Study the drawing (mm; zero at the part's minimum x, y, z) and answer. Coordinates: 2 decimals unless noted, no trailing zeros. Write each loop counter-clockwise with the first axis right and the second up, starting at its lowest first coordinate (ties: lowest second). Pieces come first, ordered by that corner, then holes. Notation, with made-up numbers: (84.5, 88.5) -> (117.5, 88.5) arc R18 ccw to (117.5, 92.5) -> close; hole circle Ø9 at (13, 5). An arc over 180 degrees is marked (long way). Answer in a Markdown table with one row per item. Add a question column.
Item 1: For a pull along X with two mould halves and no side action, classify the marked faces 1, 2 and 3 as +X half, -X half, draft (parallel to the pull), parting line (faces both ways), or undercut.
Item 2: Straight lines are drawn through the part: line 1 (Y direction, x = 6.5, z = 4.3) (1 decimal); line 2 (Y direction, x = 7.75, z = 2.7) (1 decimal); line 3 (X direction, y = 4, z = 4.3). For each, find the intervals that lie inside material, in ascending order. Write a range as from..to.
Item 3: Section D-D on x = 10 is taken. Write down the section's boundary in (y, z) (1 decimal).
Item 4: Section B-B on y = 4.25 is taken. Write down the section's boundary in (x, z) (1 decimal), then the cut area to 3 significant figures.
Item 5: Section A-A on x = 3.5 is taken. Write down the section's boundary in (y, z) (1 decimal).
Item 6: Given pin 1 Ø1 at (y, z) = (7.5, 2.5) entering from -X; pin 2 Ø1 at (x, z) = (4.5, 0.5) entering from +Y; pin 3 Ø4 at (x, y) = (5.58, 5.15) entering from -Z, each flat-ended and moving along its own axis, determine where each tip first touches the part or whether it passes through.
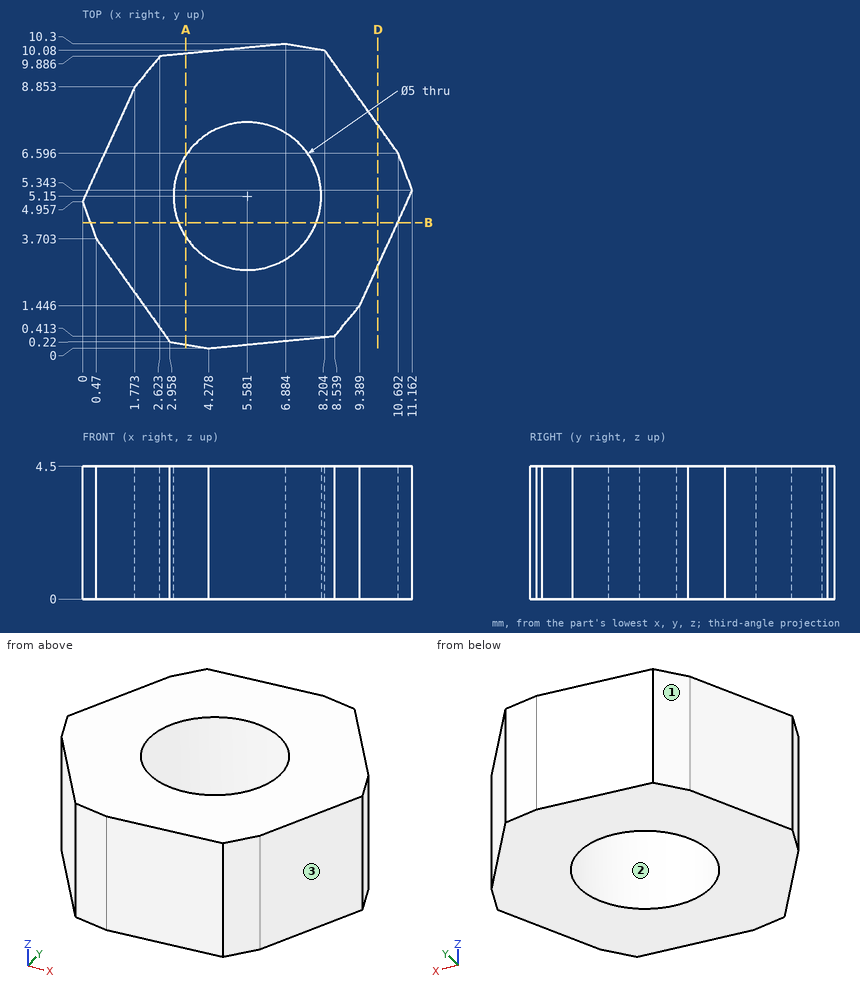
Results below:
| question | item | result |
|---|---|---|
| 1 | face 1 | -X half |
| 1 | face 2 | undercut |
| 1 | face 3 | +X half |
| 2 | line 1 | y = 0.2..2.8, 7.5..10.3 |
| 2 | line 2 | y = 0.3..3.9, 6.4..10.2 |
| 2 | line 3 | x = 0.36..3.36, 7.8..10.55 |
| 3 | outline | (2.8, 0) -> (7.6, 0) -> (7.6, 4.5) -> (2.8, 4.5) -> close |
| 4 | outline | (0.3, 0) -> (3.2, 0) -> (3.2, 4.5) -> (0.3, 4.5) -> close; (7.9, 0) -> (10.7, 0) -> (10.7, 4.5) -> (7.9, 4.5) -> close |
| 4 | area | 25.8 mm2 |
| 5 | outline | (0.1, 0) -> (3.8, 0) -> (3.8, 4.5) -> (0.1, 4.5) -> close; (6.5, 0) -> (10, 0) -> (10, 4.5) -> (6.5, 4.5) -> close |
| 6 | pin 1 | stops at x = 0.93 |
| 6 | pin 2 | stops at y = 10.12 |
| 6 | pin 3 | passes through |
